from build123d import *

# Parameters (mm, degrees)
TALADRO_ROSCADO_M101_D     = 8.5
TALADRO_ROSCADO_M101_DEPTH = 15
TALADRO_ROSCADO_M101_TIP   = 2.553657631
CORTAR_EXTRUIR1_DEPTH      = 5


with BuildPart() as part:
    # Sketch1 → Revolve1 (revolve)
    with BuildSketch(Plane.XY, mode=Mode.PRIVATE) as revolve1_sk:
        Polygon((0, 0), (-32.518320182, 0), (-32.518320182, 7.092937258), (-30, 8), (0, 8), align=None)
    revolve(revolve1_sk.sketch.rotate(Axis((0, 0, 0), (-1, 0, 0)), 90), axis=Axis((0, 0, 0), (-1, 0, 0)))

    # Taladro roscado M101
    with Locations(Plane(origin=(0, 0, 0), x_dir=(0, 0, -1), z_dir=(1, 0, 0))):
        with Locations((0, 0)):
            Hole(TALADRO_ROSCADO_M101_D / 2, depth=TALADRO_ROSCADO_M101_DEPTH)
            with Locations((0, 0, -(TALADRO_ROSCADO_M101_DEPTH + TALADRO_ROSCADO_M101_TIP / 2))):  # 118° drill point
                Cone(0, TALADRO_ROSCADO_M101_D / 2, TALADRO_ROSCADO_M101_TIP, mode=Mode.SUBTRACT)

    # Croquis3 → Cortar-Extruir1 (cut)
    with BuildSketch(Plane.ZY.offset(32.518320182)):
        Polygon((0, -3.156760752), (2.733835005, -1.578380376), (2.733835005, 1.578380376), (0, 3.156760752), (-2.733835005, 1.578380376), (-2.733835005, -1.578380376), align=None)
    extrude(amount=-CORTAR_EXTRUIR1_DEPTH, mode=Mode.SUBTRACT)


solid = part.part
Work out the finished part from the listing and answer in its coordinate system (mm). A direction names the side the tool comes from. Give positions to 0.01 mm unless a question says otherwise; leave off trailing zeros. Order: outer loops, then holes, each group sorted by start corner. A loop starts at its lowest first (then second) coordinate and runs counter-clockwise, first axis right, second up. Notation, with made-up numbers: (76, -34) -> (91, -34) arc R16 ccw to (91, -30) -> close; hole circle Ø2 at (29.5, -23). An arc over 180 degrees is marked (long way). Answer as a JSON object with one key per item and string values. Group by question number.
1. Flat-ended cylindrical pins translate along their axes: pin 1 Ø1 at (x, z) = (-4.5, -2) entering from -Y; pin 2 Ø2 at (x, z) = (-22.5, -4.5) entering from -Y; pin 3 Ø1.5 at (x, y) = (-10.5, 4.5) entering from -Z. Find the tip coordinate at first contact, or state that the pin passes through.
2. Section B-B on x = -20 is taken. Determine the outline of the cut face in (y, z), plus the area to 3 significant figures.
3. A tool of negligible diameter and unlimited length cuts with its end or side. For faces 1 (the flat face through (0, 3.4, -3.4)), 2 (the flat face through (-30.053, 2.379, -1.348)), 3 (the cylindrical face through (-7.605, 3.584, 2.285)), from which of +Z, -Z, +X, -X, +Y, -Y can it reach the whole face along a straight path? Write none if from no direction.
4. The mould has two halves that part along Y. Classify faces 4 (the conical face through (-32.361, 6.343, -3.299)), 5 (the flat face through (-32.518, 0, 3)), 6 (the flat face through (-30, 0, 2.734)), 7 (the flat face through (-30.053, 2.357, 1.386)): released by +Y, released by -Y, zero draft, split by the parting line, or undercut.
5. Consider line 1 along Y through (x, z) = (-5.75, 0); line 2 along Y through (x, z) = (-6, 2); line 3 along Z through (x, y) = (-6, -1.25). Determine where each line is inside the solid, lowest interval first. Write a range as [from, to].
6. Section A-A on x = -14 is taken. Determine the outline of the cut face in (y, z).
Result sheet:
{
 "1": {"pin 1": "stops at y = -7.86", "pin 2": "stops at y = -7.19", "pin 3": "stops at z = -7.07"},
 "2": {"outline": "circle Ø16 at (0, 0)", "area": "201 mm^2"},
 "3": {"face 1": "+Z, -Z, +X, +Y, -Y", "face 2": "-X", "face 3": "+X"},
 "4": {"face 4": "split by the parting line", "face 5": "zero draft", "face 6": "undercut", "face 7": "undercut"},
 "5": {"line 1": "y = [-8, -4.25], [4.25, 8]", "line 2": "y = [-7.75, -3.75], [3.75, 7.75]", "line 3": "z = [-7.9, -4.06], [4.06, 7.9]"},
 "6": {"outline": "circle Ø16 at (0, 0); hole circle Ø8.5 at (0, 0)"}
}
